Geometry check sheet. Reference: the model listing, model coordinates, mm. A direction names the side the tool comes from. Coordinates: 2 decimals unless noted, no trailing zeros.
Solid Edge part; units mm, degrees
sketch "Sketch1" plane through (0, 0, 0) normal (0, 0, 1) x (1, 0, 0)
  line L0 (40, -40) -> (40, 40)
  line L1 (40, 40) -> (-40, 40)
  line L2 (-40, 40) -> (-40, -40)
  line L3 (-40, -40) -> (40, -40)
extrude "Protrusion1" add sketch "Sketch1" along normal blind 530
extrude "Extrusionsausschnitt_1" [suppressed]
sketch "Sketch2" plane through (40, 0, 350) normal (1, 0, 0) x (0, 0, 1)
  circle A0 centre (50, 90) radius 60
  circle A1 centre (50, 90) radius 40
extrude "Protrusion2" add sketch "Sketch2" against normal up to vertex (80 mm away)
sketch "Sketch3" plane through (40, -55, 350) normal (1, 0, 0) x (0, 0, 1)
  line L0 (-10, 5) -> (-40, 5)
  line L1 (-40, 5) -> (-40, -15)
  line L2 (-40, -15) -> (26.1282, -15)
  line L3 (26.1282, -15) -> (-10, 35)
  line L4 (-10, 35) -> (-10, 5)
extrude "Protrusion3" add sketch "Sketch3" against normal up to vertex (80 mm away)
hole "Bohrung_1" at (0, -60, 325) direction (0, 1, 0) diameter 10 depth 30 tip angle 118 counterbore diameter 15 counterbore depth 8.8
mirror "Mirror1" [suppressed]
sketch "Sketch4" plane through (0, 0, 530) normal (0, 0, 1) x (-1, 0, 0)
  circle A0 centre (0, 0) radius 5
extrude "Extrusionsausschnitt_2" cut sketch "Sketch4" against normal blind 36.6109
sketch "Sketch5" plane through (0, 0, 530) normal (0, 0, 1) x (1, 0, 0)
  line L0 (28.5, -25.15) -> (40, -25.15)
  line L1 (40, -25.15) -> (40, -14.85)
  line L2 (40, -14.85) -> (28.5, -14.85)
  line L3 (28.5, -14.85) -> (28.5, -25.15)
  line L4 (28.5, 14.85) -> (40, 14.85)
  line L5 (40, 14.85) -> (40, 25.15)
  line L6 (40, 25.15) -> (28.5, 25.15)
  line L7 (28.5, 25.15) -> (28.5, 14.85)
extrude "Cutout1" cut sketch "Sketch5" against normal up to vertex (530 mm away)
sketch "Sketch6" plane through (0, 0, 530) normal (0, 0, 1) x (1, 0, 0)
  line L0 (-86.4024, -164.9595) -> (86.4024, -164.9595)
  line L1 (86.4024, -164.9595) -> (86.4024, -40)
  line L2 (86.4024, -40) -> (-86.4024, -40)
  line L3 (-86.4024, -40) -> (-86.4024, -164.9595)
extrude "Extrusionsausschnitt_4" cut sketch "Sketch6" against normal blind 227.9971
mirror "Mirror2" about plane through (-6.1475, 6.1475, 8.6939) normal (0.7071, 0.7071, 0) of "Cutout1"
mirror "Mirror3" about plane through (0, 0, 0) normal (1, 0, 0) of "Cutout1"
mirror "Mirror4" about plane through (0, 0, 0) normal (0, -1, 0) of "Mirror2"
hole "Bohrung_2" at (-34, -34, 0) direction (0, 0, 1) diameter 4.917 depth 35 tip angle 118 thread major 6 thread length 30
hole "Hole1" at (34, -34, 0) direction (0, 0, 1) diameter 4.917 depth 35 tip angle 118 thread major 6 thread length 30
hole "Hole2" at (34, 34, 0) direction (0, 0, 1) diameter 4.917 depth 35 tip angle 118 thread major 6 thread length 30
hole "Hole3" at (-34, 34, 0) direction (0, 0, 1) diameter 4.917 depth 35 tip angle 118 thread major 6 thread length 30
hole "Hole4" at (-20, -20, 0) direction (0, 0, 1) diameter 4.917 depth 35 tip angle 118 thread major 6 thread length 30
hole "Hole5" at (20, -20, 0) direction (0, 0, 1) diameter 4.917 depth 35 tip angle 118 thread major 6 thread length 30
hole "Hole6" at (20, 20, 0) direction (0, 0, 1) diameter 4.917 depth 35 tip angle 118 thread major 6 thread length 30
hole "Hole7" at (-20, 20, 0) direction (0, 0, 1) diameter 4.917 depth 35 tip angle 118 thread major 6 thread length 30
hole "Bohrung_6" at (-34, 34, 530) direction (0, 0, -1) diameter 4.917 depth 35 tip angle 118 thread major 6 thread length 30
hole "Hole8" at (-34, -34, 530) direction (0, 0, -1) diameter 4.917 depth 35 tip angle 118 thread major 6 thread length 30
hole "Hole9" at (34, 34, 530) direction (0, 0, -1) diameter 4.917 depth 35 tip angle 118 thread major 6 thread length 30
hole "Hole10" at (34, -34, 530) direction (0, 0, -1) diameter 4.917 depth 35 tip angle 118 thread major 6 thread length 30
hole "Hole11" at (-20, -20, 530) direction (0, 0, -1) diameter 4.917 depth 35 tip angle 118 thread major 6 thread length 30
hole "Hole12" at (-20, 20, 530) direction (0, 0, -1) diameter 4.917 depth 35 tip angle 118 thread major 6 thread length 30
hole "Hole13" at (20, 20, 530) direction (0, 0, -1) diameter 4.917 depth 35 tip angle 118 thread major 6 thread length 30
hole "Hole14" at (20, -20, 530) direction (0, 0, -1) diameter 4.917 depth 35 tip angle 118 thread major 6 thread length 30
1. Gauge pin test, flat ends, axial feed: pin 1 Ø5 at (x, y) = (0.5, -2) entering from +Z; pin 2 Ø8 at (x, z) = (-19.5, 203) entering from +Y; pin 3 Ø3 at (y, z) = (-19, 327) entering from +X. Record the tip position at first contact, or that the pin passes through.
Computed values:
pin 1: stops at z = 493.39
pin 2: stops at y = 28.5
pin 3: stops at x = 28.5
2. Draft check along X on faces 1 (the flat face through (20, 28.5, 269)), 2 (the flat face through (-28.5, -20, 269)), 3 (the flat face through (32, -40, 261)). Enter one of: released by +X, released by -X, zero draft, split by the parting line, or undercut.
Computed values:
face 1: undercut
face 2: released by -X
face 3: zero draft
3. Thickness scan on line 1 along X through (y, z) = (-36, 325); line 2 along Y through (x, z) = (36, 94.5); line 3 along X through (y, z) = (20, 24.5). Record the ranges inside material, lowest first.
Computed values:
line 1: x = -40 to -25.15, -14.85 to -5, 5 to 14.85, 25.15 to 40
line 2: y = -40 to -25.15, -14.85 to 14.85, 25.15 to 40
line 3: x = -28.5 to -22.46, -17.54 to 17.54, 22.46 to 28.5
4. Access from +Z, -Z, +X, -X, +Y, -Y to the whole of each face (thin tool, end or side, straight path). Record for faces 4 (the flat face through (0, 0, 493.389)), 5 (the flat face through (-14.85, 34, 269)), 6 (the flat face through (34, -14.85, 269)), 7 (the flat face through (-20, -28.5, 269)).
Computed values:
face 4: +Z
face 5: +Z, -Z, +Y
face 6: +Z, -Z, +X
face 7: +Z, -Z, -Y
